Here's how the part is built. I have some questions about the finished solid (model axes, mm). Face numbers are marked on the shaded views. A direction names the side the tool comes from. Round coordinates to 2 decimals unless told otherwise and drop trailing zeros. Write each loop counter-clockwise with the first axis right and the second up, starting at its lowest first coordinate (ties: lowest second). Pieces come first, ordered by that corner, then holes. Notation, with made-up numbers: M 77.5,70.25 L 100.5,70.25 A15 cw 100.5,88.25 Z; hole C 66,-38.5 d1. An arc over 180 degrees is marked long. Write item = value, one per line. Start each with the question number.
(1) I need wall thicknesses on line 1 along Z through (x, y) = (-4, 3.5); line 2 along X through (y, z) = (4.35, -2.5); line 3 along Z through (x, y) = (4.25, 5.3). Which ranges of each line are inside material? Lowest first, please.
(2) If we mould it in two halves opening along Z, with no side actions, what happens to the marked faces 4, 5, 6 and 7? For each: released by +Z, released by -Z, zero draft, split by the parting line, or undercut.
(3) On a 3-axis mill with a long thin cutter (end or side, diameter ignored), from which of +Z, -Z, +X, -X, +Y, -Y can I reach the whole of each face in a straight line? I mean the marked faces 1, 2 and 3. Say none if no direction works.
(4) I want a section at A-A (y = 2.9). List the corners of the cut face in (x, z) for me, and give its area (3 significant figures).
(5) I want a section at D-D (y = 0.4). List the corners of the cut face in (x, z) for me.
(6) I want a section at B-B (x = 0). List the corners of the cut face in (y, z) for me, and give its area (3 significant figures).
(7) I want a section at C-C (z = -2.5). List the corners of the cut face in (x, y) for me, and give its area (3 significant figures).
(8) Will these pins go through, and if not, where does the flat tip stop? pin 1 Ø1.6 at (x, z) = (0, 5) entering from +Y; pin 2 Ø1.6 at (x, z) = (-2.5, 3.5) entering from +Y.
```python
from build123d import *

# Parameters (mm, degrees)
SKETCH1_W           = 10
SKETCH1_H           = 13
BOSS_EXTRUDE1_DEPTH = 2
SKETCH2_W           = 10
SKETCH2_H           = 2
BOSS_EXTRUDE2_DEPTH = 2.5
FILLET1_R           = 2
FILLET2_R           = 0.5
SKETCH3_W           = 10
SKETCH3_H           = 8.5
BOSS_EXTRUDE3_DEPTH = 4
CUT_EXTRUDE1_REACH  = 12.161
SKETCH4_R           = 2.15
FILLET3_R           = 0.5
FILLET4_R           = 0.5


with BuildPart() as part:
    # Sketch1 → Boss-Extrude1 (new body)
    with BuildSketch(Plane(origin=(0, 0, 0), x_dir=(1, 0, 0), z_dir=(0, 1, 0))):
        Rectangle(SKETCH1_W, SKETCH1_H)
    extrude(amount=BOSS_EXTRUDE1_DEPTH)

    # Sketch2 → Boss-Extrude2 (add)
    with BuildSketch(Plane(origin=(0, 2, 0), x_dir=(1, 0, 0), z_dir=(0, 1, 0))):
        with Locations((0, -5.5)):
            Rectangle(SKETCH2_W, SKETCH2_H)
    extrude(amount=BOSS_EXTRUDE2_DEPTH)

    # Fillet1
    fillet1_edges = [part.edges().sort_by_distance(p)[0] for p in [
        (0, 0, 6.5),
    ]]
    fillet(fillet1_edges, radius=FILLET1_R)

    # Fillet2
    fillet2_edges = [part.edges().sort_by_distance(p)[0] for p in [
        (0, 4.5, 6.5),
    ]]
    fillet(fillet2_edges, radius=FILLET2_R)

    # Sketch3 → Boss-Extrude3 (add)
    with BuildSketch(Plane(origin=(0, 2, 0), x_dir=(1, 0, 0), z_dir=(0, 1, 0))):
        with Locations((0, 2.25)):
            Rectangle(SKETCH3_W, SKETCH3_H)
    extrude(amount=BOSS_EXTRUDE3_DEPTH)

    # Sketch4 → Cut-Extrude1 (cut, up to next)
    with BuildSketch(Plane(origin=(0, 6, 0), x_dir=(1, 0, 0), z_dir=(0, 1, 0)), mode=Mode.PRIVATE) as cut_extrude1_sk1:
        with Locations(Location((0, 2.5, 0), (0, 0, 270))):
            Circle(SKETCH4_R)
    cut_extrude1_tool1 = extrude(cut_extrude1_sk1.sketch, amount=-CUT_EXTRUDE1_REACH, mode=Mode.PRIVATE) & part.part
    add(cut_extrude1_tool1.solids().sort_by_distance((0, 6, -2.5))[0], mode=Mode.SUBTRACT)

    # Fillet3
    fillet3_edges = [part.edges().sort_by_distance(p)[0] for p in [
        (0, 2, 4.5),
        (0, 2, 2),
        (-5, 6, -2.25),
        (0, 6, 2),
        (5, 6, -2.25),
        (0, 6, -6.5),
        (-5, 3, -6.5),
        (5, 3, -6.5),
    ]]
    fillet(fillet3_edges, radius=FILLET3_R)

    # Fillet4
    fillet4_edges = [part.edges().sort_by_distance(p)[0] for p in [
        (0, 6, -4.65),
    ]]
    fillet(fillet4_edges, radius=FILLET4_R)


solid = part.part
```
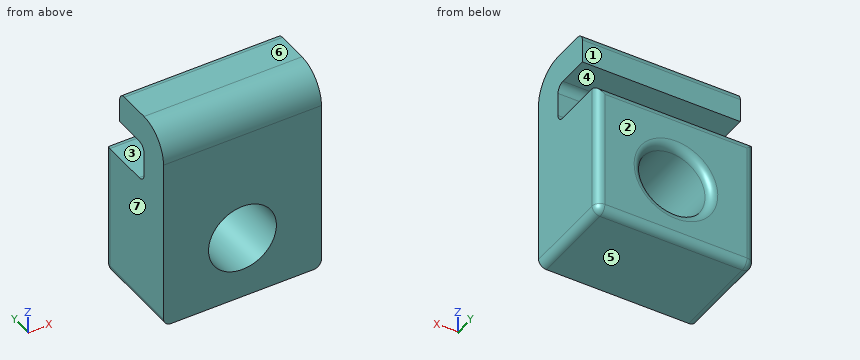
Returned:
q1.line_1 = -6.5 to 2, 4.5 to 6.5
q1.line_2 = -5 to -2.15, 2.15 to 5
q1.line_3 = -6.5 to 2
q2.face_4 = undercut
q2.face_5 = released by -Z
q2.face_6 = released by +Z
q2.face_7 = zero draft
q3.face_1 = +Z, +X, -X, +Y
q3.face_2 = +Z, -Z, +X, -X, +Y
q3.face_3 = +X, -X, +Y
q4.outline = M -5,-6 A0.5 ccw -4.5,-6.5 L 4.5,-6.5 A0.5 ccw 5,-6 L 5,2 L -5,2 Z; M -5,4.5 L 5,4.5 L 5,6.5 L -5,6.5 Z; hole C 0,-2.5 d4.3
q4.area = 90.4 mm²
q5.outline = M -5,-6 A0.5 ccw -4.5,-6.5 L 4.5,-6.5 A0.5 ccw 5,-6 L 5,5.7 L -5,5.7 Z; hole C 0,-2.5 d4.3
q6.outline = M 0,-6.5 L 5.5,-6.5 A0.5 ccw 6,-6 L 6,-5.15 A0.5 ccw 5.5,-4.65 L 0,-4.65 Z; M 0,-0.35 L 5.5,-0.35 A0.5 ccw 6,0.15 L 6,1.5 A0.5 ccw 5.5,2 L 2.5,2 A0.5 cw 2,2.5 L 2,4 A0.5 cw 2.5,4.5 L 4.5,4.5 L 4.5,6 A0.5 ccw 4,6.5 L 2,6.5 A2 ccw 0,4.5 Z
q6.area = 38.2 mm²
q7.outline = M -5,0 L -2.15,0 L -2.15,5.5 A0.5 ccw -2.65,6 L -4.5,6 A0.5 ccw -5,5.5 Z; M 2.15,0 L 5,0 L 5,5.5 A0.5 ccw 4.5,6 L 2.65,6 A0.5 ccw 2.15,5.5 Z
q7.area = 34.0 mm²
q8.pin_1 = 4.5
q8.pin_2 = 2.1
